```python
from build123d import *

# Parameters (mm, degrees)
SKETCH1_W           = 52.6
SKETCH1_H           = 11
SKETCH2_R           = 5
BOSS_EXTRUDE1_DEPTH = 1.35
SKETCH3_R           = 3.5
BOSS_EXTRUDE2_DEPTH = 1.8
SKETCH4_R           = 2
BOSS_EXTRUDE3_DEPTH = 11.7
CUT_EXTRUDE1_REACH  = 71.221
HOLE1_D             = 1.95
HOLE1_DEPTH         = 6.5
HOLE2_D             = 1.95
HOLE2_DEPTH         = 6.5
HOLE3_D             = 1.95
HOLE3_DEPTH         = 6.5
HOLE4_D             = 7
HOLE4_DEPTH         = 6.4
HOLE5_D             = 2.1
HOLE5_DEPTH         = 3
HOLE6_D             = 2.1
HOLE6_DEPTH         = 3
HOLE7_D             = 2.1
HOLE7_DEPTH         = 3
SKETCH25_R          = 11
BOSS_EXTRUDE4_DEPTH = 36.83
SKETCH26_R          = 12
SKETCH26_R_2        = 8
CUT_EXTRUDE2_DEPTH  = 6


with BuildPart() as part:
    # Sketch1 → Revolve1 (revolve)
    with BuildSketch(Plane.XY, mode=Mode.PRIVATE) as revolve1_sk:
        with Locations((26.3, 5.5)):
            Rectangle(SKETCH1_W, SKETCH1_H)
    revolve(revolve1_sk.sketch.rotate(Axis((0, 0, 0), (1, 0, 0)), 270), axis=Axis((0, 0, 0), (1, 0, 0)))

    # Sketch2 → Boss-Extrude1 (add)
    with BuildSketch(Plane.ZY):
        with Locations(Location((0, 0, 0), (0, 0, 180))):
            Circle(SKETCH2_R)
    extrude(amount=BOSS_EXTRUDE1_DEPTH)

    # Sketch3 → Boss-Extrude2 (add)
    with BuildSketch(Plane.ZY.offset(1.35)):
        Circle(SKETCH3_R)
    extrude(amount=BOSS_EXTRUDE2_DEPTH)

    # Sketch4 → Boss-Extrude3 (add)
    with BuildSketch(Plane.ZY.offset(3.15)):
        Circle(SKETCH4_R)
    extrude(amount=BOSS_EXTRUDE3_DEPTH)

    # Cut-Extrude1: up to this plane
    cut_extrude1_end = Plane(origin=(-3.675, 0, 3.675), z_dir=(0.707106781186547, 0, -0.707106781186548))
    # Sketch6 → Cut-Extrude1 (cut, up to the surface)
    with BuildSketch(Plane.ZY.offset(14.85), mode=Mode.PRIVATE) as cut_extrude1_sk1:
        with BuildLine():
            Line((1.5, 1.322875656), (1.5, -1.322875656))
            ThreePointArc((1.5, -1.322875656), (2, 0), (1.5, 1.322875656))
        make_face()
    cut_extrude1_tool1 = split(extrude(cut_extrude1_sk1.sketch, amount=-CUT_EXTRUDE1_REACH, mode=Mode.PRIVATE), bisect_by=cut_extrude1_end, keep=Keep.BOTH, mode=Mode.PRIVATE)
    add(cut_extrude1_tool1.solids().sort_by_distance((-14.85, 0, 1.702311))[0], mode=Mode.SUBTRACT)

    # Hole1
    with Locations(Plane.ZY):
        with Locations((7, 0)):
            Hole(HOLE1_D / 2, depth=HOLE1_DEPTH)

    # Hole2
    with Locations(Plane.ZY):
        with Locations((-3.5, -6.062177826)):
            Hole(HOLE2_D / 2, depth=HOLE2_DEPTH)

    # Hole3
    with Locations(Plane.ZY):
        with Locations((-3.5, 6.062177826)):
            Hole(HOLE3_D / 2, depth=HOLE3_DEPTH)

    # Hole4
    with Locations(Plane(origin=(52.6, 0, 0), x_dir=(0, 0, -1), z_dir=(1, 0, 0))):
        with Locations((0, 0)):
            Hole(HOLE4_D / 2, depth=HOLE4_DEPTH)

    # Hole5
    with Locations(Plane(origin=(52.6, 0, 0), x_dir=(0, 0, -1), z_dir=(1, 0, 0))):
        with Locations((-8.5, 0)):
            Hole(HOLE5_D / 2, depth=HOLE5_DEPTH)

    # Hole6
    with Locations(Plane(origin=(52.6, 0, 0), x_dir=(0, 0, -1), z_dir=(1, 0, 0))):
        with Locations((4.25, -7.361215932)):
            Hole(HOLE6_D / 2, depth=HOLE6_DEPTH)

    # Hole7
    with Locations(Plane(origin=(52.6, 0, 0), x_dir=(0, 0, -1), z_dir=(1, 0, 0))):
        with Locations((4.25, 7.361215932)):
            Hole(HOLE7_D / 2, depth=HOLE7_DEPTH)

    # Sketch25 → Boss-Extrude4 (add)
    with BuildSketch(Plane(origin=(52.6, 0, 0), x_dir=(0, 0, -1), z_dir=(1, 0, 0))):
        Circle(SKETCH25_R)
    extrude(amount=BOSS_EXTRUDE4_DEPTH)

    # Sketch26 → Cut-Extrude2 (cut)
    with BuildSketch(Plane(origin=(89.43, 0, 0), x_dir=(0, 0, -1), z_dir=(1, 0, 0))):
        Circle(SKETCH26_R)
        Circle(SKETCH26_R_2, mode=Mode.SUBTRACT)
    extrude(amount=-CUT_EXTRUDE2_DEPTH, mode=Mode.SUBTRACT)


solid = part.part
```
The model under review builds one solid part; all positions refer to its coordinate system, in mm. A direction names the side the tool comes from. Round coordinates to 2 decimals unless told otherwise and drop trailing zeros. Loops run counter-clockwise (first coordinate to the right, second up) from the corner with the lowest first, then second, coordinate; pieces in that order, holes last. Notation, with made-up numbers: M -21.5,83.25 L 31.5,83.25 A16 ccw 31.5,113.25 Z; hole C 77,20 d7. An arc over 180 degrees is marked long. Write item = value, one per line.
Item 1: Insertion check: P1, Ø0.6, axis at y = 6, z = -3.5, coming from the -X side; P2, Ø0.6, axis at y = 0, z = 9, coming from the +X side; P3, Ø1.3, axis at y = -7.36, z = -4.25, coming from the -X side. Each pin has a flat end and moves straight along its axis. Give the tip position at first contact, or say it passes through.
Return value:
P1 = 6.5
P2 = 83.43
P3 = 0
Item 2: Machinability: for faces 5 (the cylindrical face through (86.47, -7.81, 1.73)), 6 (the flat face through (52.6, 0, 0)), 7 (the cylindrical face through (3.296, 0.043, 7.974)), which of the approach directions +Z, -Z, +X, -X, +Y, -Y give a long, thin tool a straight path to every point of the face, cutting with its end or side? Answer none if there is none.
Return value:
face_5 = +X
face_6 = none
face_7 = -X
Item 3: For line 1 (Y direction, x = 5.25, z = -3.5); line 2 (X direction, y = 2.75, z = -2); line 3 (X direction, y = 3, z = -8.25), list the stretches that pass through material, from the lowest coordinate up. Write a range as [from, to].
Return value:
line_1 = [-10.43, -7.04], [-5.09, 5.09], [7.04, 10.43]
line_2 = [-3.15, 46.2], [52.6, 89.43]
line_3 = [0, 83.43]
Item 4: Take a section at A-A on y = 0. State how many separate pieces and enclosed holes the cut face has, then the cut area to 3 significant figures.
Return value:
separate_pieces = 1
enclosed_holes = 2
area = 1,940 mm2
Item 5: The part is to be moulded in two halves that separate along Z. For faces 1 (the flat face through (89.43, 0, 0)), 2 (the cylindrical face through (51.08, 0.32, 9.5)), 3 (the flat face through (-10, 0, 1.5)), 4 (the cylindrical face through (-2.237, -1.341, 3.233)), say which applies: released by +Z, released by -Z, zero draft, split by the parting line, or undercut.
Return value:
face_1 = zero draft
face_2 = undercut
face_3 = released by +Z
face_4 = split by the parting line
Item 6: Take a section at B-B on x = 11.5. Write out the cut boundary in (y, z), then the cut area to 3 significant figures.
Return value:
outline = C 0,0 d22
area = 380 mm2
Item 7: Take a section at C-C on x = 1. Write out the cut boundary in (y, z) (3 decimals), then the cut area to 3 significant figures.
Return value:
outline = C 0,0 d22; hole C -6.062,-3.5 d1.95; hole C 0,7 d1.95; hole C 6.062,-3.5 d1.95
area = 371 mm2
